from build123d import *

# Parameters (mm, degrees)
SKETCH2_R           = 34
BOSS_EXTRUDE1_DEPTH = 10
SKETCH3_R           = 29.8
CUT_EXTRUDE1_DEPTH  = 50.112116631
SKETCH4_W           = 1.8
SKETCH4_H           = 2.8
BOSS_EXTRUDE2_DEPTH = 10
CIRPATTERN1_COUNT   = 10
SKETCH5_W           = 2.5
SKETCH5_H           = 1
CUT_EXTRUDE2_DEPTH  = 50.112116631
CIRPATTERN3_COUNT   = 30


with BuildPart() as part:
    # Sketch2 → Boss-Extrude1 (new body)
    with BuildSketch(Plane.XY):
        Circle(SKETCH2_R)
    extrude(amount=BOSS_EXTRUDE1_DEPTH)

    # Sketch3 → Cut-Extrude1 (cut, through all)
    with BuildSketch(Plane.XY):
        Circle(SKETCH3_R)
    extrude(amount=CUT_EXTRUDE1_DEPTH, mode=Mode.SUBTRACT)

    # Sketch4 → Boss-Extrude2 (add)
    with BuildSketch(Plane.XY):
        with Locations((0, 29.8)):
            Rectangle(SKETCH4_W, SKETCH4_H)
    boss_extrude2 = extrude(amount=BOSS_EXTRUDE2_DEPTH)

    # CirPattern1: Boss-Extrude2 ×10 about axis
    cirpattern1_axis = Axis((0, 0, 0), (0, 0, 1))
    for i in range(1, CIRPATTERN1_COUNT):
        add(boss_extrude2.rotate(cirpattern1_axis, i * 360 / CIRPATTERN1_COUNT))

    # Sketch5 → Cut-Extrude2 (cut, through all)
    with BuildSketch(Plane.XY):
        with Locations((0, 34)):
            Rectangle(SKETCH5_W, SKETCH5_H)
    cut_extrude2 = extrude(amount=CUT_EXTRUDE2_DEPTH, mode=Mode.SUBTRACT)

    # CirPattern3: Cut-Extrude2 ×30 about axis
    cirpattern3_axis = Axis((0, 0, 0), (0, 0, 1))
    for i in range(1, CIRPATTERN3_COUNT):
        add(cut_extrude2.rotate(cirpattern3_axis, i * 360 / CIRPATTERN3_COUNT), mode=Mode.SUBTRACT)


solid = part.part
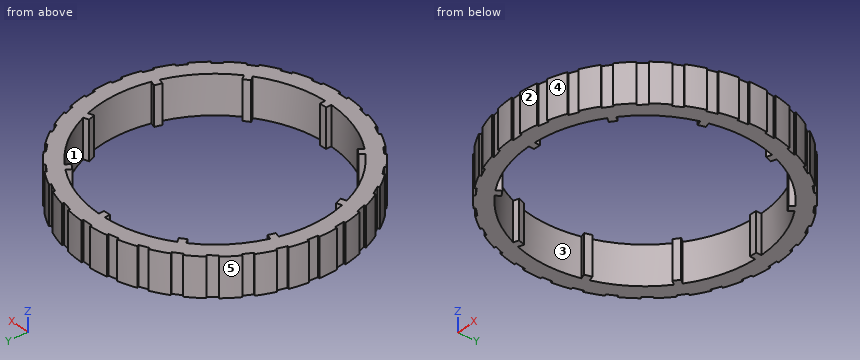
CAD build for the part. Positions are in the model's coordinates, mm. Face numbers are marked on the shaded views. A direction names the side the tool comes from. Coordinates: 2 decimals unless noted, no trailing zeros. Write each loop counter-clockwise with the first axis right and the second up, starting at its lowest first coordinate (ties: lowest second). Pieces come first, ordered by that corner, then holes. Notation, with made-up numbers: M 17.5,42 L 75.5,42 A30 cw 75.5,73 Z; hole C 26.25,50.25 d10. An arc over 180 degrees is marked long. Return JSON: item names as keys, results as strings.
Item 1: Probe line 1 (X direction, y = -23, z = 2.5); line 2 (Y direction, x = 10, z = 8.75); line 3 (Y direction, x = -22.5, z = 9). List the from-to ranges inside material, lowest first. Write a range as from..to.
Findings below:
{"line 1": "x = -24.37..-18.95, -17.82..-16.66, 16.66..17.82, 18.95..24.37", "line 2": "y = -32.5..-28.07, 28.07..32.5", "line 3": "y = -25.49..-19.54, 19.54..25.49"}
Item 2: Which spindle directions (+Z, -Z, +X, -X, +Y, -Y) get a long thin tool onto all of the face, cutting with end or side? Do the marked faces 1 and 2. Say none if no direction does.
Findings below:
{"face 1": "+Z, -Z", "face 2": "+Z, -Z, +X, -Y"}
Item 3: Two-plate mould, pull along Y, no slides. Class the marked faces 3, 4 and 5: +Y half, -Y half, draft (parallel to the pull), parting line (faces both ways), or undercut.
Findings below:
{"face 3": "undercut", "face 4": "-Y half", "face 5": "+Y half"}
Item 4: Slice it at A-A, the plane y = -19. Write the cut outline in (x, z), and give its area (3 significant figures).
Findings below:
{"outline": "M -28.2,0 L -22.96,0 L -22.96,10 L -28.2,10 Z; M 22.96,0 L 28.2,0 L 28.2,10 L 22.96,10 Z", "area": "105 mm2"}
Item 5: Slice it at B-B, the plane x = 4. Write the cut outline in (y, z).
Findings below:
{"outline": "M -33.76,0 L -29.53,0 L -29.53,10 L -33.76,10 Z; M 29.53,0 L 33.76,0 L 33.76,10 L 29.53,10 Z"}
Item 6: Drop flat-ended pins along their axis: pin 1 Ø0.9 at (x, z) = (0, 6.5) entering from -Y; pin 2 Ø0.7 at (y, z) = (-29, 4.5) entering from -X; pin 3 Ø2 at (y, z) = (11, 4) entering from +X; pin 4 Ø3 at (x, z) = (0, 3) entering from +Y. Give the stop position or say it passes through.
Findings below:
{"pin 1": "stops at y = -33.5", "pin 2": "stops at x = -18.31", "pin 3": "stops at x = 31.97", "pin 4": "stops at y = 33.98"}
